Check sheet for the modelled part. Datum: model origin and axes. Units: mm. Round coordinates to 2 decimals unless told otherwise and drop trailing zeros. Order: outer loops, then holes, each group sorted by start corner. A loop starts at its lowest first (then second) coordinate and runs counter-clockwise, first axis right, second up. Notation, with made-up numbers: (-23.5, 73.25) -> (32.5, 73.25) arc R19 cw to (32.5, 84.25) -> close; hole circle Ø2 at (38.5, -36). An arc over 180 degrees is marked (long way). Use CSV: the item, a comma, the result in double quotes.
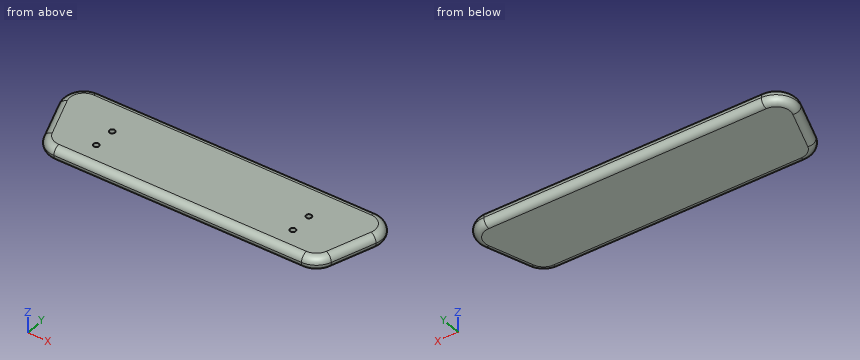
```python
from build123d import *

# Parameters (mm, degrees)
EXTRUDE_1_DEPTH     = 10
FILLET_1_R          = 15
FILLET_2_R          = 5
SKETCH_2_R          = 2
CUT_EXTRUDE_1_DEPTH = 7.5


with BuildPart() as part:
    # 草圖1 → 填料-伸長1 (new body)
    with BuildSketch(Plane.XY):
        Polygon((-123.946188341, 3.497757848), (-102.699073989, -56.502242152), (94.806697307, -56.502242152), (116.053811659, 3.497757848), align=None)
    extrude(amount=EXTRUDE_1_DEPTH)

    # 圓角1
    fillet_1_edges = [part.edges().sort_by_distance(p)[0] for p in [
        (116.053811659, 3.497757848, 5),
        (94.806697307, -56.502242152, 5),
        (-102.699073989, -56.502242152, 5),
        (-123.946188341, 3.497757848, 5),
    ]]
    fillet(fillet_1_edges, radius=FILLET_1_R)

    # 圓角2
    fillet_2_edges = [part.edges().sort_by_distance(p)[0] for p in [
        (107.078925905, -2.845064302, 10),
        (103.657146356, -31.509345041, 10),
        (92.862923252, -53.75186548, 10),
        (-3.946188341, -56.502242152, 10),
        (-100.755299934, -53.75186548, 10),
        (-111.549523037, -31.509345041, 10),
        (-114.971302586, -2.845064302, 10),
        (-3.946188341, 3.497757848, 10),
        (-114.971302586, -2.845064302, 0),
        (-111.549523037, -31.509345041, 0),
        (-100.755299934, -53.75186548, 0),
        (-3.946188341, -56.502242152, 0),
        (92.862923252, -53.75186548, 0),
        (103.657146356, -31.509345041, 0),
        (107.078925905, -2.845064302, 0),
        (-3.946188341, 3.497757848, 0),
    ]]
    fillet(fillet_2_edges, radius=FILLET_2_R - 0.0001)  # a hair under: the kernel refuses the full size

    # 草圖2 → 除料-伸長1 (cut)
    with BuildSketch(Plane.XY.offset(10)):
        with Locations((-73.946188341, -23.502242152)):
            Circle(SKETCH_2_R)
        with Locations((-73.946188341, -39.502242152)):
            Circle(SKETCH_2_R)
        with Locations(Location((66.053811659, -39.502242152, 0), (0, 0, 180))):
            Circle(SKETCH_2_R)
        with Locations(Location((66.053811659, -23.502242152, 0), (0, 0, 180))):
            Circle(SKETCH_2_R)
    extrude(amount=-CUT_EXTRUDE_1_DEPTH, mode=Mode.SUBTRACT)


solid = part.part
```
Q1. Go/stop test with flat-tipped pins: pin 1 (3 mm diameter, centred on y = -32, z = 4.5, fed in from -X); pin 2 (5 mm diameter, centred on x = 47.5, z = 1.5, fed in from -Y); pin 3 (5 mm diameter, centred on x = 79, z = 2, fed in from -Y). Record where each tip stops, or that it passes through.
Result sheet:
pin 1,"stops at x = -111.89"
pin 2,"stops at y = -56.4"
pin 3,"stops at y = -56.48"
Q2. Scan lines: L1, parallel to X at y = -25, z = 8.75; L2, parallel to X at y = -39, z = 3; L3, parallel to Z at x = 44.5, y = -52. Record each from-to range of solid material in increasing order.
Result sheet:
L1,"x = -112.06 to -75.27, -72.62 to 64.73, 67.38 to 104.17"
L2,"x = -108.45 to -75.88, -72.01 to 64.12, 67.99 to 100.56"
L3,"z = 0.02 to 9.98"
Q3. Sectioned sample at A-A, the plane z = 8.25. Enter the section's corners in (x, y).
Result sheet:
outline,"(-115.73, -16.11) -> (-105.11, -46.11) arc R13.8 ccw to (-92.1, -55.3) -> (84.21, -55.3) arc R13.8 ccw to (97.21, -46.11) -> (107.84, -16.11) arc R13.8 ccw to (94.83, 2.3) -> (-102.72, 2.3) arc R13.8 ccw to start; hole circle Ø4 at (-73.95, -39.5); hole circle Ø4 at (-73.95, -23.5); hole circle Ø4 at (66.05, -39.5); hole circle Ø4 at (66.05, -23.5)"
